```python
from build123d import *

# Parameters (mm, degrees)
SKETCH1_W                                  = 115
SKETCH1_H                                  = 115
BOSS_EXTRUDE1_DEPTH                        = 37.5
SKETCH3_R                                  = 3.15
CUT_EXTRUDE2_DEPTH                         = 80
MIRROR1_AT_THE_SECOND_PLANE_COPY_1_SKETC_R = 3.15
MIRROR1_AT_THE_SECOND_PLANE_COPY_1_DEPTH   = 80
FILLET1_R                                  = 10
CUT_EXTRUDE3_DEPTH                         = 80
CUT_EXTRUDE6_DEPTH                         = 80
FILLET2_R                                  = 2.5
FILLET3_R                                  = 10
SKETCH9_W                                  = 85
SKETCH9_H                                  = 61
CUT_EXTRUDE7_DEPTH                         = 130
SKETCH10_W                                 = 61
SKETCH10_H                                 = 85
CUT_EXTRUDE8_DEPTH                         = 120
SKETCH12_R                                 = 6.5
CUT_EXTRUDE9_DEPTH                         = 80
SKETCH13_R                                 = 1.75
CUT_EXTRUDE10_DEPTH                        = 80
CIRPATTERN1_COUNT                          = 3
SKETCH14_R                                 = 3.25
CUT_EXTRUDE11_DEPTH                        = 4
CIRPATTERN2_COUNT                          = 3
MIRROR4_COPY_1_SKETCH_R                    = 3.25
MIRROR4_COPY_1_DEPTH                       = 4
MIRROR4_COPY_2_SKETCH_R                    = 3.25
MIRROR4_COPY_2_DEPTH                       = 4
SKETCH17_R                                 = 4
CUT_EXTRUDE12_DEPTH                        = 30
CIRPATTERN3_COUNT                          = 4
SKETCH18_W                                 = 7
SKETCH18_H                                 = 20
SKETCH18_W_2                               = 20
SKETCH18_H_2                               = 7
BOSS_EXTRUDE3_DEPTH                        = 2


with BuildPart() as part:
    # Sketch1 → Boss-Extrude1 (new, symmetric)
    with BuildSketch(Plane.XY):
        Rectangle(SKETCH1_W, SKETCH1_H)
    extrude(amount=BOSS_EXTRUDE1_DEPTH, both=True)

    # Sketch3 → Cut-Extrude2 (cut)
    with BuildSketch(Plane.XY.offset(37.5)):
        with Locations((-48, 48)):
            Circle(SKETCH3_R)
    cut_extrude2 = extrude(amount=-CUT_EXTRUDE2_DEPTH, mode=Mode.SUBTRACT)

    # Mirror1: Cut-Extrude2 across plane
    add(cut_extrude2.mirror(Plane.ZX), mode=Mode.SUBTRACT)

    # Mirror1 at the second plane: Cut-Extrude2 across plane
    add(cut_extrude2.mirror(Plane(origin=(0, 0, 0), x_dir=(0, 0, 1), z_dir=(1, 0, 0))), mode=Mode.SUBTRACT)

    # Mirror1 at the second plane copy 1 sketc → Mirror1 at the second plane copy 1 (cut)
    with BuildSketch(Plane(origin=(0, 0, 37.5), x_dir=(-1, 0, 0), z_dir=(0, 0, 1))):
        with Locations((-48, 48)):
            Circle(MIRROR1_AT_THE_SECOND_PLANE_COPY_1_SKETC_R)
    extrude(amount=-MIRROR1_AT_THE_SECOND_PLANE_COPY_1_DEPTH, mode=Mode.SUBTRACT)

    # Fillet1
    fillet1_edges = [part.edges().sort_by_distance(p)[0] for p in [
        (-57.5, 57.5, 0),
        (57.5, 57.5, 0),
        (57.5, -57.5, 0),
        (-57.5, -57.5, 0),
    ]]
    fillet(fillet1_edges, radius=FILLET1_R)

    # Sketch5 → Cut-Extrude3 (cut)
    with BuildSketch(Plane.XY.offset(37.5)):
        Polygon((-40, 47.5), (-25, 47.5), (25, 47.5), (40, 47.5), (25, 32.5), (-25, 32.5), align=None)
    cut_extrude3 = extrude(amount=-CUT_EXTRUDE3_DEPTH, mode=Mode.SUBTRACT)

    # Mirror2: Cut-Extrude3 across plane
    add(cut_extrude3.mirror(Plane.ZX), mode=Mode.SUBTRACT)

    # Sketch8 → Cut-Extrude6 (cut)
    with BuildSketch(Plane.XY.offset(37.5)):
        Polygon((47.5, 25), (47.5, 40), (32.5, 25), (32.5, -25), (47.5, -40), (47.5, -25), align=None)
    cut_extrude6 = extrude(amount=-CUT_EXTRUDE6_DEPTH, mode=Mode.SUBTRACT)

    # Mirror3: Cut-Extrude6 across plane
    add(cut_extrude6.mirror(Plane(origin=(0, 0, 0), x_dir=(0, 0, 1), z_dir=(1, 0, 0))), mode=Mode.SUBTRACT)

    # Fillet2
    fillet2_edges = [part.edges().sort_by_distance(p)[0] for p in [
        (47.5, 40, 0),
        (47.5, -40, 0),
        (-47.5, 40, 0),
        (-47.5, -40, 0),
        (40, 47.5, 0),
        (-40, 47.5, 0),
        (40, -47.5, 0),
        (-40, -47.5, 0),
    ]]
    fillet(fillet2_edges, radius=FILLET2_R)

    # Fillet3
    fillet3_edges = [part.edges().sort_by_distance(p)[0] for p in [
        (32.5, 25, 0),
        (32.5, -25, 0),
        (-32.5, 25, 0),
        (-32.5, -25, 0),
        (25, 32.5, 0),
        (-25, 32.5, 0),
        (-25, -32.5, 0),
        (25, -32.5, 0),
    ]]
    fillet(fillet3_edges, radius=FILLET3_R)

    # Sketch9 → Cut-Extrude7 (cut)
    with BuildSketch(Plane(origin=(0, 57.5, 0), x_dir=(1, 0, 0), z_dir=(0, 1, 0))):
        Rectangle(SKETCH9_W, SKETCH9_H)
    extrude(amount=-CUT_EXTRUDE7_DEPTH, mode=Mode.SUBTRACT)

    # Sketch10 → Cut-Extrude8 (cut)
    with BuildSketch(Plane(origin=(57.5, 0, 0), x_dir=(0, 0, -1), z_dir=(1, 0, 0))):
        Rectangle(SKETCH10_W, SKETCH10_H)
    extrude(amount=-CUT_EXTRUDE8_DEPTH, mode=Mode.SUBTRACT)

    # Sketch12 → Cut-Extrude9 (cut)
    with BuildSketch(Plane.XY.offset(37.5)):
        Circle(SKETCH12_R)
    extrude(amount=-CUT_EXTRUDE9_DEPTH, mode=Mode.SUBTRACT)

    # Sketch13 → Cut-Extrude10 (cut)
    with BuildSketch(Plane.XY.offset(37.5)):
        with Locations((0, 12)):
            Circle(SKETCH13_R)
    cut_extrude10 = extrude(amount=-CUT_EXTRUDE10_DEPTH, mode=Mode.SUBTRACT)

    # CirPattern1: Cut-Extrude10 ×3 about axis
    cirpattern1_axis = Axis((0, 0, 0), (0, 0, 1))
    for i in range(1, CIRPATTERN1_COUNT):
        add(cut_extrude10.rotate(cirpattern1_axis, i * 360 / CIRPATTERN1_COUNT), mode=Mode.SUBTRACT)

    # Sketch14 → Cut-Extrude11 (cut)
    with BuildSketch(Plane.XY.offset(37.5)):
        with Locations((0, 12)):
            Circle(SKETCH14_R)
    cut_extrude11 = extrude(amount=-CUT_EXTRUDE11_DEPTH, mode=Mode.SUBTRACT)

    # CirPattern2: Cut-Extrude11 ×3 about axis
    cirpattern2_axis = Axis((0, 0, 0), (0, 0, 1))
    for i in range(1, CIRPATTERN2_COUNT):
        add(cut_extrude11.rotate(cirpattern2_axis, i * 360 / CIRPATTERN2_COUNT), mode=Mode.SUBTRACT)

    # Mirror4: Cut-Extrude11 across plane
    add(cut_extrude11.mirror(Plane.XY), mode=Mode.SUBTRACT)

    # Mirror4 copy 1 sketch → Mirror4 copy 1 (cut)
    with BuildSketch(Plane(origin=(0, 0, -37.5), x_dir=(-0.4999999999999998, 0.8660254037844387, 0), z_dir=(0, 0, -1))):
        with Locations((0, -12)):
            Circle(MIRROR4_COPY_1_SKETCH_R)
    extrude(amount=-MIRROR4_COPY_1_DEPTH, mode=Mode.SUBTRACT)

    # Mirror4 copy 2 sketch → Mirror4 copy 2 (cut)
    with BuildSketch(Plane(origin=(0, 0, -37.5), x_dir=(-0.5000000000000004, -0.8660254037844384, 0), z_dir=(0, 0, -1))):
        with Locations((0, -12)):
            Circle(MIRROR4_COPY_2_SKETCH_R)
    extrude(amount=-MIRROR4_COPY_2_DEPTH, mode=Mode.SUBTRACT)

    # Sketch17 → Cut-Extrude12 (cut, symmetric)
    with BuildSketch(Plane.XY):
        with Locations((-48, 48)):
            Circle(SKETCH17_R)
    cut_extrude12 = extrude(amount=CUT_EXTRUDE12_DEPTH, both=True, mode=Mode.SUBTRACT)

    # CirPattern3: Cut-Extrude12 ×4 about axis
    cirpattern3_axis = Axis((0, 0, 0), (0, 0, 1))
    for i in range(1, CIRPATTERN3_COUNT):
        add(cut_extrude12.rotate(cirpattern3_axis, i * 360 / CIRPATTERN3_COUNT), mode=Mode.SUBTRACT)

    # Sketch18 → Boss-Extrude3 (add)
    with BuildSketch(Plane.XY.offset(-30.5)):
        with Locations((-29, 0)):
            Rectangle(SKETCH18_W, SKETCH18_H)
        with Locations((29, 0)):
            Rectangle(SKETCH18_W, SKETCH18_H)
        with Locations((0, -29)):
            Rectangle(SKETCH18_W_2, SKETCH18_H_2)
    boss_extrude3 = extrude(amount=BOSS_EXTRUDE3_DEPTH)

    # Mirror5: Boss-Extrude3 across plane
    add(boss_extrude3.mirror(Plane.XY))


solid = part.part
```
The listing builds one solid part. Answer for the finished solid, in the listing's coordinates (mm). A direction names the side the tool comes from. Coordinates: 2 decimals unless noted, no trailing zeros. Loops run counter-clockwise (first coordinate to the right, second up) from the corner with the lowest first, then second, coordinate; pieces in that order, holes last. Notation, with made-up numbers: (63.5, 62.25) - (119.5, 62.25) arc R26 ccw to (119.5, 82.25) - close; hole circle Ø7 at (80, 43.5). An arc over 180 degrees is marked (long way). Write item = value, one per line.
1) Section A-A (z = 26) is taken. Determine the outline of the cut face in (x, y).
Responses:
outline = (-57.5, -47.5) arc R10 ccw to (-47.5, -57.5) - (-42.5, -57.5) - (-42.5, -42.5) - (-57.5, -42.5) - close; (-57.5, 42.5) - (-42.5, 42.5) - (-42.5, 57.5) - (-47.5, 57.5) arc R10 ccw to (-57.5, 47.5) - close; (42.5, -57.5) - (47.5, -57.5) arc R10 ccw to (57.5, -47.5) - (57.5, -42.5) - (42.5, -42.5) - close; (42.5, 42.5) - (57.5, 42.5) - (57.5, 47.5) arc R10 ccw to (47.5, 57.5) - (42.5, 57.5) - close; hole circle Ø8 at (-48, -48); hole circle Ø8 at (-48, 48); hole circle Ø8 at (48, -48); hole circle Ø8 at (48, 48)
2) Which of the six approach directions +Z, -Z, +X, -X, +Y, -Y give full straight-line access (tool end or side, diameter ignored) to faces 3 (the face through (-42.5, 50, 0)), 4 (the face through (-45, -46, -30)), 5 (the face through (-36.26, -45.99, 33.95))?
Responses:
face_3 = +Y, -Y
face_4 = none
face_5 = +Z, -Z
3) Each of these flat-tipped pins is pushed along its axis until it touches: P1, Ø4.5, axis at x = 49.5, z = -1, coming from the +Y side; P2, Ø1.6, axis at x = 29, z = -29.5, coming from the -Y side; P3, Ø0.6, axis at x = -30.5, z = 29.5, coming from the +Y side; P4, Ø1, axis at x = -4.5, z = 29.5, coming from the +Y side. Where does it stop, or does it pass through?
Responses:
P1 = 57.5
P2 = -10
P3 = 10
P4 = -25.5
4) Section B-B (y = 0) is taken. Count the separate pieces of the cut face and the enclosed holes in it, plus the area to 3 significant figures.
Responses:
separate_pieces = 8
enclosed_holes = 0
area = 1,060 mm^2
5) Determine the mould class of faces 1 (the face through (-1, -12, 37.5)), 2 (the face through (39.4, 31.9, 34)) for opening direction Y: pulls with the +Y half, pulls with the -Y half, needs draft (parallel to the pull), parting line crosses it, or undercut.
Responses:
face_1 = needs draft
face_2 = undercut
6) Find the intervals of material crossed by line 1 along Y through (x, z) = (-48, -33.75); line 2 along Y through (x, z) = (0, 36); line 3 along Z through (x, y) = (52.5, -36), in increasing order.
Responses:
line_1 = -57.49 to -51.15, -44.85 to 44.85, 51.15 to 57.49
line_2 = -57.5 to -47.5, -32.5 to -6.5, 6.5 to 8.75, 15.25 to 32.5, 47.5 to 57.5
line_3 = -37.5 to -30.5, 30.5 to 37.5
